Read the model definition and answer for the solid it produces. Units are mm, in the model's axes. A direction names the side the tool comes from. Coordinates: 2 decimals unless noted, no trailing zeros. Loops run counter-clockwise (first coordinate to the right, second up) from the corner with the lowest first, then second, coordinate; pieces in that order, holes last. Notation, with made-up numbers: (3, 12.5) -> (37, 12.5) arc R14 ccw to (37, 32.5) -> close; hole circle Ø1 at (67.25, 28.25). An arc over 180 degrees is marked (long way). Answer as CSV lines item,"result".
```python
from build123d import *

# Parameters (mm, degrees)
F1_R      = 1.75
F1_W      = 26
F1_H      = 19
F1_W_2    = 2.5
F1_H_2    = 2.5
F1_W_3    = 7.5
F2_DEPTH  = 4
F3_DEPTH  = 7
F4_DEPTH  = 27
F6_DEPTH  = 2.5
F8_DEPTH  = 2.5
F9_R      = 5
F10_R     = 1.3
F11_DEPTH = 25


with BuildPart() as f2:
    # F1 (on Top) → F2 (new body)
    with BuildSketch(Plane.XY):
        Polygon((34, 35), (36.5, 35), (44, 35), (44, 61.5), (85, 61.5), (85, 35), (92.5, 35), (95, 35), (95, 65), (36.5, 65), (25, 65), (25, 35), align=None)
        with Locations((30, 40)):
            Circle(F1_R, mode=Mode.SUBTRACT)
        with Locations((90, 40)):
            Circle(F1_R, mode=Mode.SUBTRACT)
        with Locations((30, 50)):
            Circle(F1_R, mode=Mode.SUBTRACT)
        with Locations((30, 60)):
            Circle(F1_R, mode=Mode.SUBTRACT)
        with Locations((90, 50)):
            Circle(F1_R, mode=Mode.SUBTRACT)
        with Locations((90, 60)):
            Circle(F1_R, mode=Mode.SUBTRACT)
        Polygon((44, 61.5), (44, 35), (51.5, 35), (51.5, 54), (77.5, 54), (77.5, 35), (85, 35), (85, 61.5), align=None)
        with Locations((64.5, 44.5)):
            Rectangle(F1_W, F1_H)
        with Locations((35.25, 33.75)):
            Rectangle(F1_W_2, F1_H_2)
        with Locations((40.25, 33.75)):
            Rectangle(F1_W_3, F1_H_2)
        Polygon((51.5, 35), (44, 35), (44, 32.5), (85, 32.5), (85, 35), (77.5, 35), align=None)
        with Locations((88.75, 33.75)):
            Rectangle(F1_W_3, F1_H_2)
        with Locations((93.75, 33.75)):
            Rectangle(F1_W_2, F1_H_2)
    extrude(amount=F2_DEPTH)

    # F1 (on Top) → F3 (join)
    with BuildSketch(Plane.XY):
        Polygon((44, 61.5), (44, 35), (51.5, 35), (51.5, 54), (77.5, 54), (77.5, 35), (85, 35), (85, 61.5), align=None)
        Polygon((51.5, 35), (44, 35), (44, 32.5), (85, 32.5), (85, 35), (77.5, 35), align=None)
    extrude(amount=F3_DEPTH)

    # F1 (on Top) → F4 (join)
    with BuildSketch(Plane.XY):
        with Locations((40.25, 33.75)):
            Rectangle(F1_W_3, F1_H_2)
        with Locations((88.75, 33.75)):
            Rectangle(F1_W_3, F1_H_2)
        with Locations((93.75, 33.75)):
            Rectangle(F1_W_2, F1_H_2)
        with Locations((35.25, 33.75)):
            Rectangle(F1_W_2, F1_H_2)
    extrude(amount=F4_DEPTH)

    # F5 (on face) → F6 (join)
    with BuildSketch(Plane.YZ.offset(95)):
        Polygon((65, 4), (35, 27), (35, 4), align=None)
    extrude(amount=-F6_DEPTH)

    # F7 (on face) → F8 (join)
    with BuildSketch(Plane(origin=(34, 0, 0), x_dir=(0, -1, 0), z_dir=(-1, 0, 0))):
        Polygon((-65, 4), (-35, 4), (-35, 27), align=None)
    extrude(amount=-F8_DEPTH)

    # F9
    f9_edges = [f2.edges().sort_by_distance(p)[0] for p in [
        (25, 35, 2),
        (25, 65, 2),
    ]]
    fillet(f9_edges, radius=F9_R)

    # F10 (on face) → F11 (cut)
    with BuildSketch(Plane.XZ.offset(-32.5)):
        with Locations((40, 22)):
            Circle(F10_R)
        with Locations((40, 12)):
            Circle(F10_R)
        with Locations((90, 12)):
            Circle(F10_R)
        with Locations((90, 22)):
            Circle(F10_R)
    extrude(amount=-F11_DEPTH, mode=Mode.SUBTRACT)


solid = f2.part
```
Q1. Find the intervals of material crossed by probe 1 along X at (y, z) = (57, 4.5); probe 2 along Z at (x, y) = (90, 34); probe 3 along Y at (x, z) = (90, 2.7), in increasing order. Write a range as [from, to].
Results:
probe 1,"x = [34, 36.5], [44, 85], [92.5, 95]"
probe 2,"z = [0, 10.7], [13.3, 20.7], [23.3, 27]"
probe 3,"y = [32.5, 38.25], [41.75, 48.25], [51.75, 58.25], [61.75, 65]"
Q2. A cutting plane is placed at D-D, the plane y = 57.5. Write down the section's boundary in (x, z), and give its area (3 significant figures).
Results:
outline,"(25, 0) -> (95, 0) -> (95, 9.75) -> (92.5, 9.75) -> (92.5, 4) -> (85, 4) -> (85, 7) -> (44, 7) -> (44, 4) -> (36.5, 4) -> (36.5, 9.75) -> (34, 9.75) -> (34, 4) -> (25, 4) -> close"
area,"432 mm²"
Q3. A cutting plane is placed at C-C, the plane z = 22. Write down the section's boundary in (x, y).
Results:
outline,"(34, 32.5) -> (38.7, 32.5) -> (38.7, 35) -> (36.5, 35) -> (36.5, 41.52) -> (34, 41.52) -> close; (41.3, 32.5) -> (44, 32.5) -> (44, 35) -> (41.3, 35) -> close; (85, 32.5) -> (88.7, 32.5) -> (88.7, 35) -> (85, 35) -> close; (91.3, 32.5) -> (95, 32.5) -> (95, 41.52) -> (92.5, 41.52) -> (92.5, 35) -> (91.3, 35) -> close"
Q4. For a pull along X with two mould halves and no side action, classify faces 5 (the face through (92.5, 43, 11)), 6 (the face through (27, 64, 2)), 7 (the face through (93.77, 50.21, 15.34)) as pulls with the +X half, pulls with the -X half, needs draft (parallel to the pull), parting line crosses it, or undercut.
Results:
face 5,"undercut"
face 6,"pulls with the -X half"
face 7,"needs draft"
Q5. A cutting plane is placed at A-A, the plane y = 50. Write down the section's boundary in (x, z).
Results:
outline,"(25, 0) -> (28.25, 0) -> (28.25, 4) -> (25, 4) -> close; (31.75, 0) -> (88.25, 0) -> (88.25, 4) -> (85, 4) -> (85, 7) -> (77.5, 7) -> (77.5, 4) -> (51.5, 4) -> (51.5, 7) -> (44, 7) -> (44, 4) -> (36.5, 4) -> (36.5, 15.5) -> (34, 15.5) -> (34, 4) -> (31.75, 4) -> close; (91.75, 0) -> (95, 0) -> (95, 15.5) -> (92.5, 15.5) -> (92.5, 4) -> (91.75, 4) -> close"
Q6. For faces 1 (the face through (64, 57, 7)), 2 (the face through (28.61, 58.94, 1.97)), 3 (the face through (40, 35, 15)), 4 (the face through (64, 45, 4)), determine the directions among +Z, -Z, +X, -X, +Y, -Y from which every point of the face is accessible in a straight line to the end or side of a thin tool.
Results:
face 1,"+Z, +Y, -Y"
face 2,"+Z, -Z"
face 3,"+Z, +Y"
face 4,"+Z"
Q7. A cutting plane is placed at B-B, the plane x = 90. Write down the section's boundary in (y, z), and give its area (4 significant figures).
Results:
outline,"(32.5, 0) -> (38.25, 0) -> (38.25, 4) -> (35, 4) -> (35, 10.7) -> (32.5, 10.7) -> close; (32.5, 13.3) -> (35, 13.3) -> (35, 20.7) -> (32.5, 20.7) -> close; (32.5, 23.3) -> (35, 23.3) -> (35, 27) -> (32.5, 27) -> close; (41.75, 0) -> (48.25, 0) -> (48.25, 4) -> (41.75, 4) -> close; (51.75, 0) -> (58.25, 0) -> (58.25, 4) -> (51.75, 4) -> close; (61.75, 0) -> (65, 0) -> (65, 4) -> (61.75, 4) -> close"
area,"132.5 mm²"
Q8. Given pin 1 Ø1 at (x, y) = (36.5, 56.5) entering from +Z; pin 2 Ø5 at (y, z) = (46, 19.5) entering from -X; pin 3 Ø3 at (x, z) = (86.5, 8) entering from +Y, each flat-ended and moving along its own axis, determine where each tip first touches the part or whether it passes through.
Results:
pin 1,"stops at z = 10.9"
pin 2,"stops at x = 34"
pin 3,"stops at y = 35"
